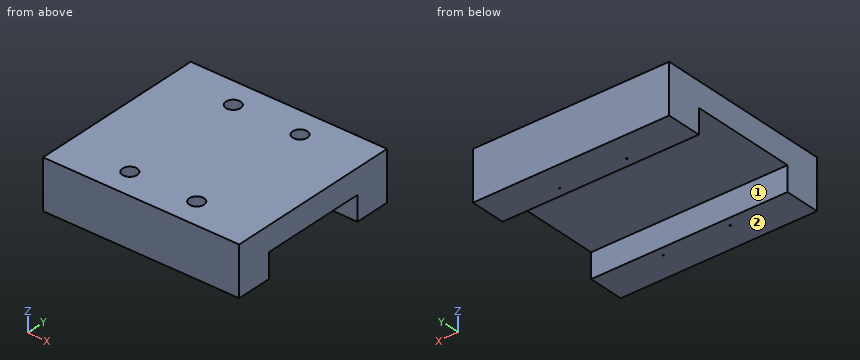
```python
from build123d import *

# Parameters (mm, degrees)
SKETCH_1_W             = 44
SKETCH_1_H             = 40
EXTRUDE_1_DEPTH        = 11
SKETCH_2_W             = 5.5
SKETCH_2_H             = 24
CUT_EXTRUDE_1_DEPTH    = 61.473134531
HOLE_WIZARD_M4_1_D     = 3.3
HOLE_WIZARD_M4_1_DEPTH = 10.1
HOLE_WIZARD_M4_1_TIP   = 0.991420021


with BuildPart() as part:
    # 草图1 → 凸台-拉伸1 (new body)
    with BuildSketch(Plane.XY):
        with Locations((22, 20)):
            Rectangle(SKETCH_1_W, SKETCH_1_H)
    extrude(amount=EXTRUDE_1_DEPTH)

    # 草图2 → 切除-拉伸1 (cut, through all)
    with BuildSketch(Plane.ZY):
        with Locations((2.75, 20)):
            Rectangle(SKETCH_2_W, SKETCH_2_H)
    extrude(amount=-CUT_EXTRUDE_1_DEPTH, mode=Mode.SUBTRACT)

    # M4 螺纹孔1
    with Locations(Plane.XY.offset(11)):
        with Locations((14.5, 34), (29.5, 34), (14.5, 6), (29.5, 6)):
            Hole(HOLE_WIZARD_M4_1_D / 2, depth=HOLE_WIZARD_M4_1_DEPTH)
            with Locations((0, 0, -(HOLE_WIZARD_M4_1_DEPTH + HOLE_WIZARD_M4_1_TIP / 2))):  # 118° drill point
                Cone(0, HOLE_WIZARD_M4_1_D / 2, HOLE_WIZARD_M4_1_TIP, mode=Mode.SUBTRACT)


solid = part.part
```
Part model, mm, in its own coordinate system. Face numbers are marked on the shaded views. A direction names the side the tool comes from. Round coordinates to 2 decimals unless told otherwise and drop trailing zeros. Loops run counter-clockwise (first coordinate to the right, second up) from the corner with the lowest first, then second, coordinate; pieces in that order, holes last.
Item 1: Cut at A-A, the plane z = 3.75. Give the cut face in (x, y), then the cut area to 3 significant figures.
Item 2: Cut at D-D, the plane y = 29.5. Give the cut face in (x, z).
Item 3: Drill centre lines: line 1 (X direction, y = 34, z = 6.5); line 2 (Y direction, x = 14.5, z = 9.25); line 3 (Y direction, x = 14.5, z = 4). Where is each one in solid material? Low to high.
Item 4: Cut at B-B, the plane x = 27. Give the cut face in (y, z).
Item 5: 3-axis set-ups, long thin cutter, end or side, ignore diameter. For the marked faces 1 and 2: which of +Z, -Z, +X, -X, +Y, -Y reach the whole face in a straight line?
Item 6: Cut at C-C, the plane z = 9. Give the cut face in (x, y), then the cut area to 3 significant figures.
Item 7: Drop flat-ended pins along their axis: P1, Ø5, axis at x = 23.5, y = 17, coming from the -Z side; P2, Ø2.5, axis at x = 29.5, y = 34, coming from the +Z side. Give the stop position or say it passes through.
A:
1. outline: (0, 0) - (44, 0) - (44, 8) - (0, 8) - close; (0, 32) - (44, 32) - (44, 40) - (0, 40) - close; hole circle Ø3.3 at (14.5, 6); hole circle Ø3.3 at (14.5, 34); hole circle Ø3.3 at (29.5, 6); hole circle Ø3.3 at (29.5, 34)
1. area: 670 mm2
2. outline: (0, 5.5) - (44, 5.5) - (44, 11) - (0, 11) - close
3. line 1: x = 0 to 12.85, 16.15 to 27.85, 31.15 to 44
3. line 2: y = 0 to 4.35, 7.65 to 32.35, 35.65 to 40
3. line 3: y = 0 to 4.35, 7.65 to 8, 32 to 32.35, 35.65 to 40
4. outline: (0, 0) - (8, 0) - (8, 5.5) - (32, 5.5) - (32, 0) - (40, 0) - (40, 11) - (0, 11) - close
5. face 1: -Z, +X, -X
5. face 2: -Z, +X, -X, +Y, -Y
6. outline: (0, 0) - (44, 0) - (44, 40) - (0, 40) - close; hole circle Ø3.3 at (14.5, 6); hole circle Ø3.3 at (14.5, 34); hole circle Ø3.3 at (29.5, 6); hole circle Ø3.3 at (29.5, 34)
6. area: 1,730 mm2
7. P1: stops at z = 5.5
7. P2: stops at z = 0.66
